from build123d import *

# Parameters (mm, degrees)
F1_DEPTH = 20


with BuildPart() as f1:
    # F0 (on Front) → F1 (new body)
    with BuildSketch(Plane.XZ):
        with BuildLine():
            ThreePointArc((-5.940089, 16.035642), (-9.847151, 17.890695), (-12.573514, 14.533122))
            ThreePointArc((-12.573514, 14.533122), (-17.076209, 13.600936), (-16.769733, 9.012985))
            ThreePointArc((-16.769733, 9.012985), (-19.818074, 5.778568), (-17.235455, 2.161398))
            Line((-17.235455, 2.161398), (-15.416807, 2.161398))
            ThreePointArc((-15.416807, 2.161398), (-15.341632, 2.182526), (-15.266946, 2.205325))
            ThreePointArc((-15.266946, 2.205325), (-15.257997, 2.183331), (-15.248898, 2.161398))
            Line((-15.248898, 2.161398), (0.599075, 2.161398))
            Line((0.599075, 2.161398), (1.466817, 2.161398))
            Line((1.466817, 2.161398), (2.837026, 2.161398))
            Line((2.837026, 2.161398), (4.730743, 2.161398))
            ThreePointArc((4.730743, 2.161398), (4.926621, 3.811509), (5.861452, 5.185307))
            ThreePointArc((5.861452, 5.185307), (5.64524, 5.301362), (5.421428, 5.401982))
            ThreePointArc((5.421428, 5.401982), (5.727707, 5.506425), (6.023032, 5.638709))
            ThreePointArc((6.023032, 5.638709), (6.081628, 5.525636), (6.1443, 5.41477))
            ThreePointArc((6.1443, 5.41477), (8.177085, 6.085562), (10.220286, 5.447202))
            ThreePointArc((10.220286, 5.447202), (12.947827, 6.708886), (15.648336, 5.390333))
            ThreePointArc((15.648336, 5.390333), (17.392275, 6.035167), (19.220387, 5.695841))
            ThreePointArc((19.220387, 5.695841), (23.005934, 6.355332), (25.115261, 3.143474))
            ThreePointArc((25.115261, 3.143474), (25.098006, 2.796362), (25.046411, 2.452672))
            ThreePointArc((25.046411, 2.452672), (25.622278, 2.433805), (26.193437, 2.509672))
            ThreePointArc((26.193437, 2.509672), (26.316013, 2.331581), (26.449351, 2.161398))
            Line((26.449351, 2.161398), (31.823543, 2.161398))
            ThreePointArc((31.823543, 2.161398), (32.032567, 2.438734), (32.213077, 2.735419))
            ThreePointArc((32.213077, 2.735419), (32.508273, 2.429381), (32.838403, 2.161398))
            Line((32.838403, 2.161398), (36.281702, 2.161398))
            Line((36.281702, 2.161398), (36.911824, 2.161398))
            Line((36.911824, 2.161398), (46.510172, 2.161398))
            ThreePointArc((46.510172, 2.161398), (46.844985, 2.554338), (47.118356, 2.992253))
            ThreePointArc((47.118356, 2.992253), (47.25325, 2.566504), (47.441262, 2.161398))
            Line((47.441262, 2.161398), (53.58981, 2.161398))
            ThreePointArc((53.58981, 2.161398), (53.609488, 2.198076), (53.628728, 2.234985))
            ThreePointArc((53.628728, 2.234985), (53.6808, 2.197712), (53.733544, 2.161398))
            Line((53.733544, 2.161398), (57.650192, 2.161398))
            ThreePointArc((57.650192, 2.161398), (57.711534, 2.203767), (57.771959, 2.247433))
            ThreePointArc((57.771959, 2.247433), (57.830262, 2.203804), (57.889461, 2.161398))
            Line((57.889461, 2.161398), (61.906458, 2.161398))
            ThreePointArc((61.906458, 2.161398), (61.914706, 2.167195), (61.922937, 2.173016))
            ThreePointArc((61.922937, 2.173016), (61.930484, 2.167197), (61.938047, 2.161398))
            Line((61.938047, 2.161398), (66.189721, 2.161398))
            ThreePointArc((66.189721, 2.161398), (67.462375, 4.105018), (67.237666, 6.417336))
            ThreePointArc((67.237666, 6.417336), (69.30512, 7.959865), (69.754252, 10.499952))
            ThreePointArc((69.754252, 10.499952), (71.331241, 15.573923), (66.076262, 16.359591))
            ThreePointArc((66.076262, 16.359591), (63.666049, 17.343961), (61.242942, 16.391769))
            ThreePointArc((61.242942, 16.391769), (59.374481, 17.015844), (57.464914, 16.531934))
            ThreePointArc((57.464914, 16.531934), (55.581553, 16.979922), (53.748163, 16.358292))
            ThreePointArc((53.748163, 16.358292), (50.433059, 16.178923), (48.759147, 13.31185))
            ThreePointArc((48.759147, 13.31185), (47.671864, 14.037602), (46.394121, 14.313776))
            ThreePointArc((46.394121, 14.313776), (43.551728, 16.132472), (40.494129, 14.704908))
            ThreePointArc((40.494129, 14.704908), (38.808881, 14.966861), (37.19991, 14.401271))
            ThreePointArc((37.19991, 14.401271), (35.298822, 14.847046), (33.454766, 14.204929))
            ThreePointArc((33.454766, 14.204929), (32.831306, 14.915761), (32.040328, 15.433774))
            ThreePointArc((32.040328, 15.433774), (26.086101, 12.988903), (19.774679, 14.252293))
            ThreePointArc((19.774679, 14.252293), (19.47591, 13.831908), (19.242162, 13.372182))
            ThreePointArc((19.242162, 13.372182), (17.473764, 13.860622), (15.70123, 13.387412))
            ThreePointArc((15.70123, 13.387412), (13.055743, 14.849641), (10.257811, 13.705836))
            ThreePointArc((10.257811, 13.705836), (7.997811, 15.876464), (4.905806, 15.367808))
            ThreePointArc((4.905806, 15.367808), (3.027117, 17.230013), (0.381927, 17.24577))
            ThreePointArc((0.381927, 17.24577), (-3.077319, 18.604807), (-5.809141, 16.084784))
            ThreePointArc((-5.809141, 16.084784), (-5.874893, 16.060954), (-5.940089, 16.035642))
        make_face()
        with BuildLine():
            ThreePointArc((23.254268, 8.608952), (23.215618, 8.600301), (23.176873, 8.592087))
            ThreePointArc((23.176873, 8.592087), (23.203012, 8.614169), (23.229366, 8.635994))
            ThreePointArc((23.229366, 8.635994), (23.241782, 8.62244), (23.254268, 8.608952))
        make_face(mode=Mode.SUBTRACT)
        with BuildLine():
            ThreePointArc((24.700602, 9.348636), (24.721351, 9.353109), (24.742126, 9.357456))
            ThreePointArc((24.742126, 9.357456), (24.715987, 9.335374), (24.689633, 9.313549))
            ThreePointArc((24.689633, 9.313549), (24.630678, 9.266264), (24.570715, 9.220262))
            ThreePointArc((24.570715, 9.220262), (24.549477, 9.263361), (24.52765, 9.306164))
            ThreePointArc((24.52765, 9.306164), (24.613856, 9.3285), (24.700602, 9.348636))
        make_face(mode=Mode.SUBTRACT)
    extrude(amount=F1_DEPTH)


solid = f1.part
Can you work these out from the model? Positions are in its coordinate system, mm. Coordinates: 2 decimals unless noted, no trailing zeros. Loops run counter-clockwise (first coordinate to the right, second up) from the corner with the lowest first, then second, coordinate; pieces in that order, holes last. Notation, with made-up numbers: M -29,-14 L -1,-14 A19 cw -1,-9 Z; hole C 21,-13.5 d7. An arc over 180 degrees is marked long. Return JSON: item names as keys, results as strings. Group by question number.
Item 1: Imagine slicing it at C-C (z = 11.75). Please give me the cut outline in (x, y), and give its area (3 significant figures).
Item 2: I'm going to push a flat-ended pin straight in: pin 1 Ø1 at (y, z) = (-8, 16) entering from -X. Where does the tip first touch, or does it pass through?
Item 3: If I drill on L1, parallel to Z at x = 11, y = -7; L2, parallel to X at y = -10, z = 5.75; L3, parallel to Z at x = 34, y = -14.75, over which ranges is the centre line in solid material (lowest first)? Write a range as from..to.
Item 4: Imagine slicing it at A-A (y = -8.75). Give the number of separate pieces and of enclosed holes in the cut face, and give its area (3 significant figures).
Item 5: Thinking about a two-plate mould opening in X: for faces 1 (the cylindrical face through (22.95, -9.86, 6.38)), 2 (the flat face through (50, -10, 2.161)), which applies, released by +X, released by -X, zero draft, split by the parting line, or undercut?
Item 6: Imagine slicing it at B-B (x = 8.5). Please give me the cut outline in (y, z), and give its area (3 significant figures).
Verdict:
{
 "1": {"outline": "M -17.78,-20 L 71.26,-20 L 71.26,0 L -17.78,0 Z", "area": "1,780 mm^2"},
 "2": {"pin 1": "stops at x = -12.42"},
 "3": {"L1": "z = 6.14..14.33", "L2": "x = -19.82..6.71, 9.7..10.5, 15.32..16.28, 19.1..19.28, 23.95..67.47", "L3": "z = 2.16..14.52"},
 "4": {"separate pieces": "1", "enclosed holes": "2", "area": "1,110 mm^2"},
 "5": {"face 1": "undercut", "face 2": "zero draft"},
 "6": {"outline": "M -20,6.07 L 0,6.07 L 0,15.68 L -20,15.68 Z", "area": "192 mm^2"}
}
